Could you check a few things on this model? Use its own coordinates, in mm. Round coordinates to 2 decimals unless told otherwise and drop trailing zeros. Loops run counter-clockwise (first coordinate to the right, second up) from the corner with the lowest first, then second, coordinate; pieces in that order, holes last. Notation, with made-up numbers: (-15, -2.75) -> (14, -2.75) arc R18 cw to (14, 31.25) -> close; hole circle Ø4 at (23.5, -23.75). An arc over 180 degrees is marked (long way). Use CSV: the item, a comma, the result in double quotes. Start each with the question number.
```python
from build123d import *

# Parameters (mm, degrees)
SKETCH1_R                            = 7
SKETCH1_R_2                          = 2
BOSS_EXTRUDE1_DEPTH                  = 7
BOSS_EXTRUDE1_2_DEPTH                = 7
BOSS_EXTRUDE2_REACH                  = 136.864
BOSS_EXTRUDE2_END_RADIUS             = 7
SKETCH2_R                            = 3
BOSS_EXTRUDE2_DIRECTION_2_REACH      = 136.864
BOSS_EXTRUDE2_DIRECTION_2_END_RADIUS = 7


with BuildPart() as part:
    # Sketch1 → Boss-Extrude1 (new body)
    with BuildSketch(Plane(origin=(0, 0, 0), x_dir=(1, 0, 0), z_dir=(0, 1, 0))):
        with Locations(Location((0, 0, 0), (0, 0, 270))):
            Circle(SKETCH1_R)
        with Locations(Location((0, 0, 0), (0, 0, 270))):
            Circle(SKETCH1_R_2, mode=Mode.SUBTRACT)
    extrude(amount=BOSS_EXTRUDE1_DEPTH)



with BuildPart() as body_2:
    # Sketch1 → Boss-Extrude1 2 (new body)
    with BuildSketch(Plane(origin=(0, 0, 0), x_dir=(1, 0, 0), z_dir=(0, 1, 0))):
        with Locations(Location((150, 0, 0), (0, 0, 270))):
            Circle(SKETCH1_R)
        with Locations(Location((150, 0, 0), (0, 0, 270))):
            Circle(SKETCH1_R_2, mode=Mode.SUBTRACT)
    extrude(amount=BOSS_EXTRUDE1_2_DEPTH)


with BuildPart() as part_1:
    add(part.part)

    add(body_2.part)  # Boss-Extrude2 merges body 2
    # Boss-Extrude2: up to this cylinder (the profile starts outside it)
    boss_extrude2_end = Plane(origin=(150, 3.5, 0), z_dir=(0, -1, 0)) * Cylinder(BOSS_EXTRUDE2_END_RADIUS, 288.728, mode=Mode.PRIVATE)
    # Sketch2 → Boss-Extrude2 (add, up to the surface)
    with BuildSketch(Plane(origin=(22.5, 0, 0), x_dir=(0, 0, -1), z_dir=(1, 0, 0)), mode=Mode.PRIVATE) as boss_extrude2_sk1:
        with Locations(Location((0, 3.5, 0), (0, 0, 180))):
            Circle(SKETCH2_R)
    boss_extrude2_tool1 = extrude(boss_extrude2_sk1.sketch, amount=BOSS_EXTRUDE2_REACH, mode=Mode.PRIVATE) - boss_extrude2_end
    add(boss_extrude2_tool1.solids().sort_by_distance((22.5, 3.5, 0))[0])

    # Boss-Extrude2 direction 2: up to this cylinder (the profile starts outside it)
    boss_extrude2_direction_2_end = Plane(origin=(0, 3.5, 0), z_dir=(0, -1, 0)) * Cylinder(BOSS_EXTRUDE2_DIRECTION_2_END_RADIUS, 288.728, mode=Mode.PRIVATE)
    # Sketch2 → Boss-Extrude2 direction 2 (add, up to the surface)
    with BuildSketch(Plane(origin=(22.5, 0, 0), x_dir=(0, 0, -1), z_dir=(1, 0, 0)), mode=Mode.PRIVATE) as boss_extrude2_direction_2_sk1:
        with Locations(Location((0, 3.5, 0), (0, 0, 180))):
            Circle(SKETCH2_R)
    boss_extrude2_direction_2_tool1 = extrude(boss_extrude2_direction_2_sk1.sketch, amount=-BOSS_EXTRUDE2_DIRECTION_2_REACH, mode=Mode.PRIVATE) - boss_extrude2_direction_2_end
    add(boss_extrude2_direction_2_tool1.solids().sort_by_distance((22.5, 3.5, 0))[0])


solid = part_1.part
```
1. If I drill on L1, parallel to X at y = 4.25, z = 0; L2, parallel to X at y = 5.5, z = 0.75; L3, parallel to X at y = 1, z = -4, over which ranges is the centre line in solid material (lowest first)?
2. Suppose I cut it at D-D (x = 65.5). List the corners of the cut face in (y, z) for me, then the cut area to 3 significant figures.
3. Suppose I cut it at B-B (z = 0). List the corners of the cut face in (x, y) for me, then the cut area to 3 significant figures.
4. We'd pull the mould along Z, two halves only. Please class faces 1 (the face through (148.226, 3.451, 0.923)), 2 (the face through (2, 0, 1)), 3 (the face through (-2, 3, 0)), 4 (the face through (155.902, 3.451, 3.763)): pulls with the +Z half, pulls with the -Z half, needs draft (parallel to the pull), parting line crosses it, or undercut.
5. Suppose I cut it at C-C (y = 3.5). List the corners of the cut face in (x, z) for me, then the cut area to 3 significant figures.
6. Suppose I cut it at A-A (x = 150). List the corners of the cut face in (y, z) for me, then the cut area to 3 significant figures.
7. Will these pins go through, and if not, where does the flat tip stop? pin 1 (8 mm diameter, centred on x = 72, z = 4, fed in from +Y); pin 2 (3 mm diameter, centred on x = 0, z = 0, fed in from -Y); pin 3 (2 mm diameter, centred on x = 12, y = 4.5, fed in from +Z); pin 4 (1 mm diameter, centred on x = 66, y = 5.5, fed in from +Z).
Geometry check:
1,L1,"x = -7 to -2, 2 to 148, 152 to 157"
1,L2,"x = -6.96 to -1.85, 1.85 to 148.15, 151.85 to 156.96"
1,L3,"x = -5.74 to 5.74, 144.26 to 155.74"
2,outline,"circle Ø6 at (3.5, 0)"
2,area,"28.3 mm²"
3,outline,"(-7, 0) -> (-2, 0) -> (-2, 7) -> (-7, 7) -> close; (2, 0) -> (7, 0) -> (7, 0.5) -> (143, 0.5) -> (143, 0) -> (148, 0) -> (148, 7) -> (143, 7) -> (143, 6.5) -> (7, 6.5) -> (7, 7) -> (2, 7) -> close; (152, 0) -> (157, 0) -> (157, 7) -> (152, 7) -> close"
3,area,"956 mm²"
4,face 1,"undercut"
4,face 2,"needs draft"
4,face 3,"undercut"
4,face 4,"parting line crosses it"
5,outline,"(6.32, -3) -> (143.68, -3) arc R7 ccw (long way) to (143.68, 3) -> (6.32, 3) arc R7 ccw (long way) to start; hole circle Ø4 at (0, 0); hole circle Ø4 at (150, 0)"
5,area,"1,100 mm²"
6,outline,"(0, -7) -> (7, -7) -> (7, -2) -> (0, -2) -> close; (0, 2) -> (7, 2) -> (7, 7) -> (0, 7) -> close"
6,area,"70.0 mm²"
7,pin 1,"stops at y = 6.5"
7,pin 2,"passes through"
7,pin 3,"stops at z = 3"
7,pin 4,"stops at z = 2.6"
